For this review, take the finished solid that the model builds, in its own axes (mm). Give positions to 0.01 mm unless a question says otherwise; leave off trailing zeros. Loops run counter-clockwise (first coordinate to the right, second up) from the corner with the lowest first, then second, coordinate; pieces in that order, holes last.
```python
from build123d import *

# Parameters (mm, degrees)
SKETCH2_W           = 3.175
SKETCH2_H           = 75.333333334
BOSS_EXTRUDE1_DEPTH = 3.175
SKETCH3_W           = 3.175
SKETCH3_H           = 78.508333333
SKETCH3_W_2         = 75.333333334
SKETCH3_H_2         = 3.175
BOSS_EXTRUDE2_DEPTH = 3.175
SKETCH4_W           = 3.175
SKETCH4_H           = 78.508333333
CUT_EXTRUDE1_DEPTH  = 3.175


with BuildPart() as part:
    # Sketch2 → Boss-Extrude1 (new body)
    with BuildSketch(Plane(origin=(0, 0, 0), x_dir=(0, 0, -1), z_dir=(1, 0, 0))):
        Polygon((-113, 37.666666667), (-113, -37.666666667), (-116.175, -37.666666667), (-116.175, -116.175), (-37.666666667, -116.175), (-37.666666667, -113), (37.666666667, -113), (37.666666667, -116.175), (116.175, -116.175), (116.175, -37.666666667), (119.35, -37.666666667), (119.35, 37.666666667), (116.175, 37.666666667), (116.175, 116.175), (37.666666667, 116.175), (37.666666667, 119.35), (-37.666666667, 119.35), (-37.666666667, 116.175), (-116.175, 116.175), (-116.175, 37.666666667), align=None)
        with Locations((39.254166667, 0)):
            Rectangle(SKETCH2_W, SKETCH2_H, mode=Mode.SUBTRACT)
        with Locations((-39.254166667, 0)):
            Rectangle(SKETCH2_W, SKETCH2_H, mode=Mode.SUBTRACT)
    extrude(amount=BOSS_EXTRUDE1_DEPTH)

    # Sketch3 → Boss-Extrude2 (add)
    with BuildSketch(Plane(origin=(3.175, 0, 0), x_dir=(0, 0, -1), z_dir=(1, 0, 0))):
        with Locations((-117.7625, 76.920833334)):
            Rectangle(SKETCH3_W, SKETCH3_H)
        with Locations((-117.7625, -76.920833334)):
            Rectangle(SKETCH3_W, SKETCH3_H)
        with Locations((0, 120.9375)):
            Rectangle(SKETCH3_W_2, SKETCH3_H_2)
    extrude(amount=-BOSS_EXTRUDE2_DEPTH)

    # Sketch4 → Cut-Extrude1 (cut)
    with BuildSketch(Plane(origin=(3.175, 0, 0), x_dir=(0, 0, -1), z_dir=(1, 0, 0))):
        with Locations((114.5875, 76.920833334)):
            Rectangle(SKETCH4_W, SKETCH4_H)
        with Locations((114.5875, -76.920833334)):
            Rectangle(SKETCH4_W, SKETCH4_H)
    extrude(amount=-CUT_EXTRUDE1_DEPTH, mode=Mode.SUBTRACT)


solid = part.part
```
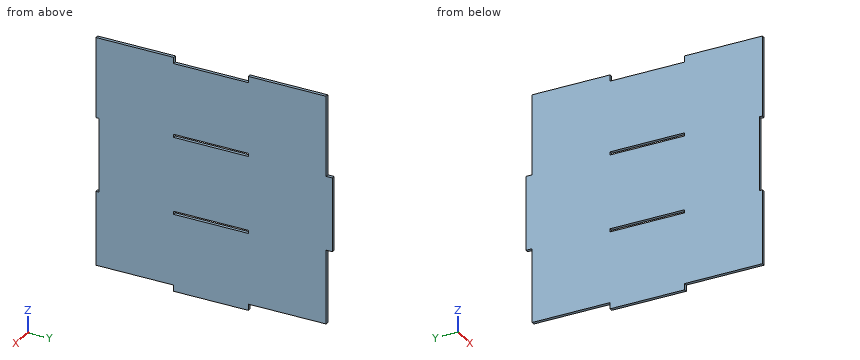
Item 1: Take a section at A-A on y = 16. Give the boundary of the cut face in (x, z) (3 decimals).
Answer:
outline: (0, -119.35) - (3.175, -119.35) - (3.175, -40.842) - (0, -40.842) - close; (0, -37.667) - (3.175, -37.667) - (3.175, 37.667) - (0, 37.667) - close; (0, 40.842) - (3.175, 40.842) - (3.175, 113) - (0, 113) - close
Item 2: Take a section at D-D on y = -77. Give the boundary of the cut face in (x, z) (3 decimals), and give its area (3 significant figures).
Answer:
outline: (0, -113) - (3.175, -113) - (3.175, 119.35) - (0, 119.35) - close
area: 738 mm2
Item 3: For L1, parallel to Z at x = 0.6, y = -15.5; L2, parallel to Y at x = 0.7, z = 38 (3 decimals); L3, parallel to Z at x = 0.8, y = -58.5, list the stretches that pass through material, from the lowest coordinate up.
Answer:
L1: z = -119.35 to -40.84, -37.67 to 37.67, 40.84 to 113
L2: y = -116.175 to -37.667, 37.667 to 116.175
L3: z = -113 to 119.35
Item 4: Clearance check with flat-ended pins moving along their axes: pin 1 Ø1.5 at (x, z) = (2.5, -95) entering from +Y (3 decimals); pin 2 Ø1 at (x, y) = (1.5, 5) entering from +Z; pin 3 Ø1 at (x, y) = (1.5, -84.5) entering from -Z; pin 4 Ø2 at (y, z) = (53, 26.5) entering from -X. State where each tip first meets the part, or that it passes through.
Answer:
pin 1: stops at y = 116.175
pin 2: stops at z = 113
pin 3: stops at z = -113
pin 4: stops at x = 0
Item 5: Take a section at B-B on x = 2.25. Give the boundary of the cut face in (y, z) (3 decimals), and give its area (3 significant figures).
Answer:
outline: (-116.175, -113) - (-37.667, -113) - (-37.667, -119.35) - (37.667, -119.35) - (37.667, -113) - (116.175, -113) - (116.175, -37.667) - (122.525, -37.667) - (122.525, 37.667) - (116.175, 37.667) - (116.175, 119.35) - (37.667, 119.35) - (37.667, 113) - (-37.667, 113) - (-37.667, 119.35) - (-116.175, 119.35) - (-116.175, 37.667) - (-113, 37.667) - (-113, -37.667) - (-116.175, -37.667) - close; hole (-37.667, -40.842) - (37.667, -40.842) - (37.667, -37.667) - (-37.667, -37.667) - close; hole (-37.667, 37.667) - (37.667, 37.667) - (37.667, 40.842) - (-37.667, 40.842) - close
area: 53,700 mm2
Item 6: Take a section at C-C on z = -70. Give the boundary of the cut face in (x, y) (3 decimals).
Answer:
outline: (0, -116.175) - (3.175, -116.175) - (3.175, 116.175) - (0, 116.175) - close
